```python
from build123d import *

# Parameters (mm, degrees)
SKETCH_1_W                  = 800
SKETCH_1_H                  = 1000
EXTRUDE_1_DEPTH             = 50
CUT_EXTRUDE_1_DEPTH         = 1079.192932642
PATTERN_LINEAR_1_COUNT      = 4
PATTERN_LINEAR_1_PITCH      = 100
PATTERN_LINEAR_1_COL_COUNT  = 3
PATTERN_LINEAR_1_COL_PITCH  = 100
FILLET_1_R                  = 50
SKETCH_5_W                  = 64
SKETCH_5_H                  = 92.5
SKETCH_5_W_2                = 92.5
SKETCH_5_H_2                = 64
CUT_EXTRUDE_2_DEPTH         = 4
HOLE_WIZARD_M30_1_D         = 26.5
HOLE_WIZARD_M30_1_DEPTH     = 70.5
HOLE_WIZARD_M30_1_TIP       = 7.961403202
HOLE_WIZARD_M8_1_D          = 6.8
HOLE_WIZARD_M8_1_DEPTH      = 19.75
HOLE_WIZARD_M8_1_TIP        = 2.042926105
HOLE_WIZARD_M8_2_AT_2_COUNT = 2
HOLE_WIZARD_M8_2_AT_2_PITCH = 44.5
HOLE_WIZARD_M8_2_AT_3_COUNT = 2
HOLE_WIZARD_M8_2_AT_3_PITCH = 86.864319487
HOLE_WIZARD_M8_2_AT_4_COUNT = 2
HOLE_WIZARD_M8_2_AT_4_PITCH = 74.6
HOLE_WIZARD_M8_3_AT_2_COUNT = 2
HOLE_WIZARD_M8_3_AT_2_PITCH = 44.5
HOLE_WIZARD_M8_3_AT_3_COUNT = 2
HOLE_WIZARD_M8_3_AT_3_PITCH = 86.864319487
HOLE_WIZARD_M8_3_AT_4_COUNT = 2
HOLE_WIZARD_M8_3_AT_4_PITCH = 74.6


with BuildPart() as part:
    # 草图1 → 凸台-拉伸1 (new body)
    with BuildSketch(Plane.XY):
        Rectangle(SKETCH_1_W, SKETCH_1_H)
    extrude(amount=EXTRUDE_1_DEPTH)

    # 草图3 → 切除-拉伸1 (cut, through all)
    with BuildSketch(Plane(origin=(0, 500, 0), x_dir=(1, 0, 0), z_dir=(0, 1, 0))):
        Polygon((-8, 0), (8, 0), (8, -13), (17.5, -13), (17.5, -25), (-17.5, -25), (-17.5, -13), (-8, -13), align=None)
    cut_extrude_1 = extrude(amount=-CUT_EXTRUDE_1_DEPTH, mode=Mode.SUBTRACT)

    # 阵列(线性)1: 切除-拉伸1 ×4
    with Locations(*[(-i * PATTERN_LINEAR_1_PITCH, 0, 0) for i in range(1, PATTERN_LINEAR_1_COUNT)]):
        add(cut_extrude_1, mode=Mode.SUBTRACT)

    # 阵列(线性)1 col: 切除-拉伸1 ×3
    with Locations(*[(i * PATTERN_LINEAR_1_COL_PITCH, 0, 0) for i in range(1, PATTERN_LINEAR_1_COL_COUNT)]):
        add(cut_extrude_1, mode=Mode.SUBTRACT)

    # 圆角1
    fillet_1_edges = [part.edges().sort_by_distance(p)[0] for p in [
        (400, -500, 25),
        (-400, -500, 25),
        (-400, 500, 25),
        (400, 500, 25),
    ]]
    fillet(fillet_1_edges, radius=FILLET_1_R)

    # 草图5 → 切除-拉伸2 (cut)
    with BuildSketch(Plane.XY.offset(50)):
        with Locations((0, 453.75)):
            Rectangle(SKETCH_5_W, SKETCH_5_H)
        with Locations((-353.75, 0)):
            Rectangle(SKETCH_5_W_2, SKETCH_5_H_2)
        with Locations((353.75, 0)):
            Rectangle(SKETCH_5_W_2, SKETCH_5_H_2)
        with Locations((0, -453.75)):
            Rectangle(SKETCH_5_W, SKETCH_5_H)
    extrude(amount=-CUT_EXTRUDE_2_DEPTH, mode=Mode.SUBTRACT)

    # M30 螺纹孔1
    with Locations(Plane.XY.offset(50)):
        with Locations((-350, 450), (350, 450), (350, -450), (-350, -450)):
            Hole(HOLE_WIZARD_M30_1_D / 2, depth=HOLE_WIZARD_M30_1_DEPTH)
            with Locations((0, 0, -(HOLE_WIZARD_M30_1_DEPTH + HOLE_WIZARD_M30_1_TIP / 2))):  # 118° drill point
                Cone(0, HOLE_WIZARD_M30_1_D / 2, HOLE_WIZARD_M30_1_TIP, mode=Mode.SUBTRACT)

    # M8 螺纹孔1
    with Locations(Plane(origin=(0, 0, 0), x_dir=(-1, 0, 0), z_dir=(0, 0, -1))):
        with Locations((-375, -165), (-375, 165)):
            Hole(HOLE_WIZARD_M8_1_D / 2, depth=HOLE_WIZARD_M8_1_DEPTH)
            with Locations((0, 0, -(HOLE_WIZARD_M8_1_DEPTH + HOLE_WIZARD_M8_1_TIP / 2))):  # 118° drill point
                Cone(0, HOLE_WIZARD_M8_1_D / 2, HOLE_WIZARD_M8_1_TIP, mode=Mode.SUBTRACT)

    # 草图12 → M8 螺纹孔2 (revolve, cut)
    with BuildSketch(Plane(origin=(-22.25, 416.45, 46), x_dir=(0, -1, 0), z_dir=(1, 0, 0))):
        Polygon((0, 0), (0, 19.792926105), (3.4, 17.75), (3.4, 0), align=None)
    hole_wizard_m8_2 = revolve(axis=Axis((-22.25, 416.45, 52.35), (0, 0, -1)), mode=Mode.SUBTRACT)

    # M8 螺纹孔2 at 2: M8 螺纹孔2 ×2
    with Locations(*[(i * HOLE_WIZARD_M8_2_AT_2_PITCH, 0, 0) for i in range(1, HOLE_WIZARD_M8_2_AT_2_COUNT)]):
        add(hole_wizard_m8_2, mode=Mode.SUBTRACT)

    # M8 螺纹孔2 at 3: M8 螺纹孔2 ×2
    with Locations(*[Vector(0.5122931977436572, 0.8588106191388054, 0) * (i * HOLE_WIZARD_M8_2_AT_3_PITCH) for i in range(1, HOLE_WIZARD_M8_2_AT_3_COUNT)]):
        add(hole_wizard_m8_2, mode=Mode.SUBTRACT)

    # M8 螺纹孔2 at 4: M8 螺纹孔2 ×2
    with Locations(*[(0, i * HOLE_WIZARD_M8_2_AT_4_PITCH, 0) for i in range(1, HOLE_WIZARD_M8_2_AT_4_COUNT)]):
        add(hole_wizard_m8_2, mode=Mode.SUBTRACT)

    # 镜向1: M8 螺纹孔2 across plane
    add(hole_wizard_m8_2.mirror(Plane.ZX), mode=Mode.SUBTRACT)

    # 镜向1 copy 1 sketch → 镜向1 copy 1 (revolve, cut)
    with BuildSketch(Plane(origin=(22.25, -416.45, 46), x_dir=(0, 1, 0), z_dir=(1, 0, 0))):
        Polygon((0, 0), (0, -19.792926105), (3.4, -17.75), (3.4, 0), align=None)
    revolve(axis=Axis((22.25, -416.45, 52.35), (0, 0, 1)), mode=Mode.SUBTRACT)

    # 镜向1 copy 2 sketch → 镜向1 copy 2 (revolve, cut)
    with BuildSketch(Plane(origin=(22.25, -491.05, 46), x_dir=(0, 1, 0), z_dir=(1, 0, 0))):
        Polygon((0, 0), (0, -19.792926105), (3.4, -17.75), (3.4, 0), align=None)
    revolve(axis=Axis((22.25, -491.05, 52.35), (0, 0, 1)), mode=Mode.SUBTRACT)

    # 镜向1 copy 3 sketch → 镜向1 copy 3 (revolve, cut)
    with BuildSketch(Plane(origin=(-22.25, -491.05, 46), x_dir=(0, 1, 0), z_dir=(1, 0, 0))):
        Polygon((0, 0), (0, -19.792926105), (3.4, -17.75), (3.4, 0), align=None)
    revolve(axis=Axis((-22.25, -491.05, 52.35), (0, 0, 1)), mode=Mode.SUBTRACT)

    # 草图14 → M8 螺纹孔3 (revolve, cut)
    with BuildSketch(Plane(origin=(-391.05, -22.25, 46), x_dir=(0, -1, 0), z_dir=(1, 0, 0))):
        Polygon((0, 0), (0, 19.792926105), (3.4, 17.75), (3.4, 0), align=None)
    hole_wizard_m8_3 = revolve(axis=Axis((-391.05, -22.25, 52.35), (0, 0, -1)), mode=Mode.SUBTRACT)

    # M8 螺纹孔3 at 2: M8 螺纹孔3 ×2
    with Locations(*[(0, i * HOLE_WIZARD_M8_3_AT_2_PITCH, 0) for i in range(1, HOLE_WIZARD_M8_3_AT_2_COUNT)]):
        add(hole_wizard_m8_3, mode=Mode.SUBTRACT)

    # M8 螺纹孔3 at 3: M8 螺纹孔3 ×2
    with Locations(*[Vector(0.8588106191388053, 0.5122931977436572, 0) * (i * HOLE_WIZARD_M8_3_AT_3_PITCH) for i in range(1, HOLE_WIZARD_M8_3_AT_3_COUNT)]):
        add(hole_wizard_m8_3, mode=Mode.SUBTRACT)

    # M8 螺纹孔3 at 4: M8 螺纹孔3 ×2
    with Locations(*[(i * HOLE_WIZARD_M8_3_AT_4_PITCH, 0, 0) for i in range(1, HOLE_WIZARD_M8_3_AT_4_COUNT)]):
        add(hole_wizard_m8_3, mode=Mode.SUBTRACT)

    # 镜向2: M8 螺纹孔3 across plane
    add(hole_wizard_m8_3.mirror(Plane(origin=(0, 0, 0), x_dir=(0, 0, 1), z_dir=(1, 0, 0))), mode=Mode.SUBTRACT)

    # 镜向2 copy 1 sketch → 镜向2 copy 1 (revolve, cut)
    with BuildSketch(Plane(origin=(391.05, 22.25, 46), x_dir=(0, -1, 0), z_dir=(-1, 0, 0))):
        Polygon((0, 0), (0, -19.792926105), (3.4, -17.75), (3.4, 0), align=None)
    revolve(axis=Axis((391.05, 22.25, 52.35), (0, 0, 1)), mode=Mode.SUBTRACT)

    # 镜向2 copy 2 sketch → 镜向2 copy 2 (revolve, cut)
    with BuildSketch(Plane(origin=(316.45, 22.25, 46), x_dir=(0, -1, 0), z_dir=(-1, 0, 0))):
        Polygon((0, 0), (0, -19.792926105), (3.4, -17.75), (3.4, 0), align=None)
    revolve(axis=Axis((316.45, 22.25, 52.35), (0, 0, 1)), mode=Mode.SUBTRACT)

    # 镜向2 copy 3 sketch → 镜向2 copy 3 (revolve, cut)
    with BuildSketch(Plane(origin=(316.45, -22.25, 46), x_dir=(0, -1, 0), z_dir=(-1, 0, 0))):
        Polygon((0, 0), (0, -19.792926105), (3.4, -17.75), (3.4, 0), align=None)
    revolve(axis=Axis((316.45, -22.25, 52.35), (0, 0, 1)), mode=Mode.SUBTRACT)


solid = part.part
```
Read the model definition and answer for the solid it produces. Units are mm, in the model's axes. A direction names the side the tool comes from. Give positions to 0.01 mm unless a question says otherwise; leave off trailing zeros. Write item = value, one per line. Start each with the question number.
Item 1: Each of these flat-tipped pins is pushed along its axis until it touches: P1, Ø2, axis at x = 10, z = 48.5, coming from the +Y side; P2, Ø11, axis at x = 22.25, y = -416.45, coming from the +Z side; P3, Ø10.5, axis at x = 1, y = -213.5, coming from the -Z side. Where does it stop, or does it pass through?
Item 2: Find the intervals of material crossed by probe 1 along Y at (x, z) = (-324.5, 47.5); probe 2 along X at (y, z) = (416.45, 34.75); probe 3 along Y at (x, z) = (22.25, 40.5), in increasing order. Write a range as [from, to].
Item 3: The mould has two halves that part along X. Classify faces 6 (the cylindrical face through (363.237, -449.417, 24.65)), 7 (the cylindrical face through (-336.763, 450.583, 24.65)), 8 (the flat face through (400, -6, 25)), 9 (the flat face through (49, 7, 0)): +X half, -X half, draft (parallel to the pull), parting line (faces both ways), or undercut.
Item 4: A tool of negligible diameter and unlimited length cuts with its end or side. For faces 1 (the flat face through (0, -453, 46)), 2 (the flat face through (-51, 7, 0)), 3 (the flat face through (353, 0, 46)), 4 (the flat face through (-100, 7, 25)), 5 (the cylindrical face through (384.964, -485.742, 25.35)), from which of +Z, -Z, +X, -X, +Y, -Y can it reach the whole face along a straight path? Write none if from no direction.
Response:
q1.P1 = 407.5
q1.P2 = 46
q1.P3 = 25
q2.probe_1 = [-500, -32], [32, 500]
q2.probe_2 = [-400, -25.65], [-18.85, 18.85], [25.65, 400]
q2.probe_3 = [-500, -494.45], [-487.65, -419.85], [-413.05, 413.05], [419.85, 487.65], [494.45, 500]
q3.face_6 = undercut
q3.face_7 = undercut
q3.face_8 = +X half
q3.face_9 = draft
q4.face_1 = +Z, -Y
q4.face_2 = -Z, +X, -X, +Y, -Y
q4.face_3 = +Z, +X
q4.face_4 = +Y, -Y
q4.face_5 = +Z, -Z, +X, -Y
